Read the model definition and answer for the solid it produces. Units are mm, in the model's axes. Face numbers are marked on the shaded views. A direction names the side the tool comes from. Coordinates: 2 decimals unless noted, no trailing zeros. Order: outer loops, then holes, each group sorted by start corner. A loop starts at its lowest first (then second) coordinate and runs counter-clockwise, first axis right, second up. Notation, with made-up numbers: (73.5, 9.5) -> (97.5, 9.5) arc R19 ccw to (97.5, 31.5) -> close; hole circle Ø2 at (43.5, 58). An arc over 180 degrees is marked (long way). Return JSON: item names as keys, results as strings. Group by question number.
```python
from build123d import *

# Parameters (mm, degrees)
SKETCH019_R     = 36
SKETCH019_R_2   = 28
SKETCH019_R_3   = 2
PAD003_DEPTH    = 4
SKETCH037_W     = 6
SKETCH037_H     = 12
PAD015_DEPTH    = 8
POCKET018_DEPTH = 8
SKETCH039_R     = 1.5
POCKET019_DEPTH = 9


with BuildPart() as part:
    # Sketch019 → Pad003 (new body)
    with BuildSketch(Plane.XY):
        Circle(SKETCH019_R)
        Circle(SKETCH019_R_2, mode=Mode.SUBTRACT)
        with Locations((-16, 27.712813)):
            Circle(SKETCH019_R_3, mode=Mode.SUBTRACT)
        with Locations((16, 27.712813)):
            Circle(SKETCH019_R_3, mode=Mode.SUBTRACT)
        with Locations((32, 0)):
            Circle(SKETCH019_R_3, mode=Mode.SUBTRACT)
        with Locations((16, -27.712813)):
            Circle(SKETCH019_R_3, mode=Mode.SUBTRACT)
        with Locations((-16, -27.712813)):
            Circle(SKETCH019_R_3, mode=Mode.SUBTRACT)
        with Locations((-32, 0)):
            Circle(SKETCH019_R_3, mode=Mode.SUBTRACT)
    extrude(amount=PAD003_DEPTH)

    # Sketch037 (on Face10 of Pad003) → Pad015 (join)
    with BuildSketch(Plane.XY.offset(4)):
        with Locations((3, 29.496479)):
            Rectangle(SKETCH037_W, SKETCH037_H)
        with Locations((3, -30)):
            Rectangle(SKETCH037_W, SKETCH037_H)
    extrude(amount=PAD015_DEPTH)

    # Sketch038 (on Face14 of Pad015) → Pocket018 (cut)
    with BuildSketch(Plane.YZ.offset(6)):
        Polygon((35.496479, 4), (34.014362, 4), (32.343197, 12), (35.496479, 12), align=None)
        Polygon((23.496479, 4), (25.836313, 4), (24.094032, 12), (23.496479, 12), align=None)
        Polygon((-24, 4), (-25.796526, 4), (-24, 12), align=None)
        Polygon((-36, 4), (-34.010136, 4), (-32.232297, 12), (-36, 12), align=None)
    extrude(amount=-POCKET018_DEPTH, mode=Mode.SUBTRACT)

    # Sketch039 (on Face10 of Pocket018) → Pocket019 (cut)
    with BuildSketch(Plane.YZ.offset(6)):
        with Locations((-29, 7.95)):
            Circle(SKETCH039_R)
        with Locations((29, 7.95)):
            Circle(SKETCH039_R)
    extrude(amount=-POCKET019_DEPTH, mode=Mode.SUBTRACT)


solid = part.part
```
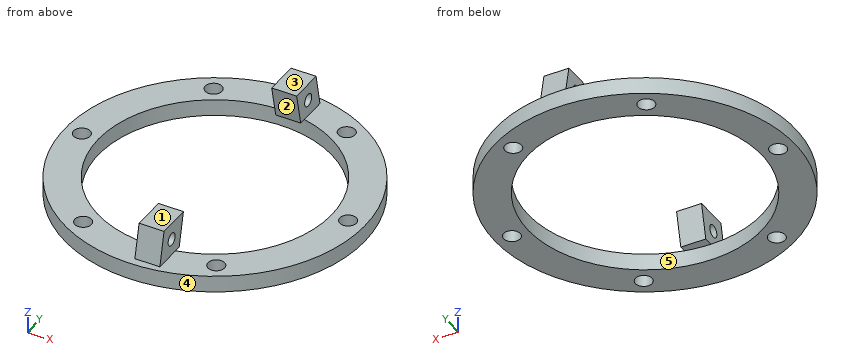
1. For a pull along X with two mould halves and no side action, classify the marked faces 3, 4 and 5 as released by +X, released by -X, zero draft, split by the parting line, or undercut.
2. Find section A-A on x = 16. Determine the outline of the cut face in (y, z).
3. Given pin 1 (2.5 mm diameter, centred on x = -16, y = -27.71, fed in from +Z); pin 2 (2.5 mm diameter, centred on y = -26.5, z = 9.5, fed in from +X); pin 3 (2.5 mm diameter, centred on y = -27, z = 10, fed in from -X); pin 4 (5 mm diameter, centred on x = 27.5, y = -14, fed in from +Z), each flat-ended and moving along its own axis, determine where each tip first touches the part or whether it passes through.
4. Which of the six approach directions +Z, -Z, +X, -X, +Y, -Y give full straight-line access (tool end or side, diameter ignored) to the marked faces 1 and 2?
5. Find section C-C on z = 11. Determine the outline of the cut face in (x, y).
6. Straight lines are drawn through the part: L1, parallel to Y at x = -1, z = 3.75; L2, parallel to Z at x = 4, y = 29; L3, parallel to Y at x = 16, z = 3.1. For each, find the intervals that lie inside material, in ascending order.
7. Find section B-B on y = -20. Determine the outline of the cut face in (x, z), and give its area (3 significant figures).
Result:
{
 "1": {"face 3": "zero draft", "face 4": "split by the parting line", "face 5": "undercut"},
 "2": {"outline": "(-32.25, 0) -> (-29.71, 0) -> (-29.71, 4) -> (-32.25, 4) -> close; (-25.71, 0) -> (-22.98, 0) -> (-22.98, 4) -> (-25.71, 4) -> close; (22.98, 0) -> (25.71, 0) -> (25.71, 4) -> (22.98, 4) -> close; (29.71, 0) -> (32.25, 0) -> (32.25, 4) -> (29.71, 4) -> close"},
 "3": {"pin 1": "through", "pin 2": "x = 6", "pin 3": "x = 0", "pin 4": "z = 4"},
 "4": {"face 1": "+Z, +X, -X, +Y, -Y", "face 2": "-Z, +X, -X"},
 "5": {"outline": "(0, -32.45) -> (6, -32.45) -> (6, -24.22) -> (0, -24.22) -> close; (0, 24.31) -> (6, 24.31) -> (6, 32.55) -> (0, 32.55) -> close"},
 "6": {"L1": "-35.99 to -27.98, 27.98 to 35.99", "L2": "0 to 6.45, 9.45 to 12", "L3": "-32.25 to -29.71, -25.71 to -22.98, 22.98 to 25.71, 29.71 to 32.25"},
 "7": {"outline": "(-29.93, 0) -> (-19.6, 0) -> (-19.6, 4) -> (-29.93, 4) -> close; (19.6, 0) -> (29.93, 0) -> (29.93, 4) -> (19.6, 4) -> close", "area": "82.7 mm^2"}
}
